Design review of the part built by this model. Coordinates are the model's own, in mm. Face numbers are marked on the shaded views. A direction names the side the tool comes from. Give positions to 0.01 mm unless a question says otherwise; leave off trailing zeros. Write each loop counter-clockwise with the first axis right and the second up, starting at its lowest first coordinate (ties: lowest second). Pieces come first, ordered by that corner, then holes.
```python
from build123d import *

# Parameters (mm, degrees)
SKETCH_1_R          = 10
SKETCH_1_R_2        = 7.5
EXTRUDE_1_DEPTH     = 80
SKETCH_2_W          = 50
SKETCH_2_H          = 20
EXTRUDE_2_DEPTH     = 70
SKETCH_3_W          = 40
SKETCH_3_H          = 20
CUT_EXTRUDE_1_DEPTH = 65
SKETCH_4_R          = 5.393818753
CUT_EXTRUDE_2_DEPTH = 159.429795178
FILLET_1_RADIUS     = 10
FILLET_1_LENGTH     = 5
FILLET_2_RADIUS     = 10
FILLET_2_LENGTH     = 5
EXTRUDE_START       = 80
SKETCH_5_R          = 7.5
EXTRUDE_3_DEPTH     = 80


with BuildPart() as part:
    # 草图1 → 凸台-拉伸1 (new body)
    with BuildSketch(Plane(origin=(0, 0, 0), x_dir=(1, 0, 0), z_dir=(0, 1, 0))):
        with Locations(Location((0, 0, 0), (0, 0, 270))):
            Circle(SKETCH_1_R)
        with Locations(Location((0, 0, 0), (0, 0, 270))):
            Circle(SKETCH_1_R_2, mode=Mode.SUBTRACT)
    extrude(amount=EXTRUDE_1_DEPTH)

    # 草图2 → 凸台-拉伸2 (add)
    with BuildSketch(Plane(origin=(0, 80, 0), x_dir=(1, 0, 0), z_dir=(0, 1, 0))):
        Rectangle(SKETCH_2_W, SKETCH_2_H)
    extrude(amount=EXTRUDE_2_DEPTH)

    # 草图3 → 切除-拉伸1 (cut)
    with BuildSketch(Plane(origin=(0, 150, 0), x_dir=(1, 0, 0), z_dir=(0, 1, 0))):
        Rectangle(SKETCH_3_W, SKETCH_3_H)
    extrude(amount=-CUT_EXTRUDE_1_DEPTH, mode=Mode.SUBTRACT)

    # 草图4 → 切除-拉伸2 (cut, through all)
    with BuildSketch(Plane.ZY.offset(25)):
        with Locations((0, 138.858219845)):
            Circle(SKETCH_4_R)
    extrude(amount=-CUT_EXTRUDE_2_DEPTH, mode=Mode.SUBTRACT)

    # 圆角1: full round fillet: the end face becomes a half cylinder, R = half its width
    fillet_1_face = Plane((-22.5, 150, 0), x_dir=(1, 0, 0), z_dir=(0, 1, 0))  # on the end face: x along it, z out of the body
    fillet_1_slab = fillet_1_face.offset(-FILLET_1_RADIUS / 2) * Box(FILLET_1_LENGTH, 2 * FILLET_1_RADIUS, FILLET_1_RADIUS, mode=Mode.PRIVATE)  # the body's end, R deep
    fillet_1_round = Plane((-22.5, 140, 0), x_dir=(0, 1, 0), z_dir=(1, 0, 0)) * Cylinder(FILLET_1_RADIUS, FILLET_1_LENGTH, mode=Mode.PRIVATE)  # its axis R under the face
    add(fillet_1_slab - fillet_1_round, mode=Mode.SUBTRACT)

    # 圆角2: full round fillet: the end face becomes a half cylinder, R = half its width
    fillet_2_face = Plane((22.5, 150, 0), x_dir=(-1, 0, 0), z_dir=(0, 1, 0))  # on the end face: x along it, z out of the body
    fillet_2_slab = fillet_2_face.offset(-FILLET_2_RADIUS / 2) * Box(FILLET_2_LENGTH, 2 * FILLET_2_RADIUS, FILLET_2_RADIUS, mode=Mode.PRIVATE)  # the body's end, R deep
    fillet_2_round = Plane((22.5, 140, 0), x_dir=(0, 1, 0), z_dir=(-1, 0, 0)) * Cylinder(FILLET_2_RADIUS, FILLET_2_LENGTH, mode=Mode.PRIVATE)  # its axis R under the face
    add(fillet_2_slab - fillet_2_round, mode=Mode.SUBTRACT)

    # 草图5 → 凸台-拉伸3 (add)
    with BuildSketch(Plane.XZ.offset(-80).offset(EXTRUDE_START)):
        Circle(SKETCH_5_R)
    extrude(amount=-EXTRUDE_3_DEPTH)

    # 草图6 → 旋转1 (revolve)
    with BuildSketch(Plane.XY):
        with BuildLine():
            Line((0, 4.111647453), (0, -10.888352547))
            ThreePointArc((0, -10.888352547), (7.5, -3.388352547), (0, 4.111647453))
        make_face()
    revolve(axis=Axis((0, 4.111647453, 0), (0, -1, 0)))


solid = part.part
```
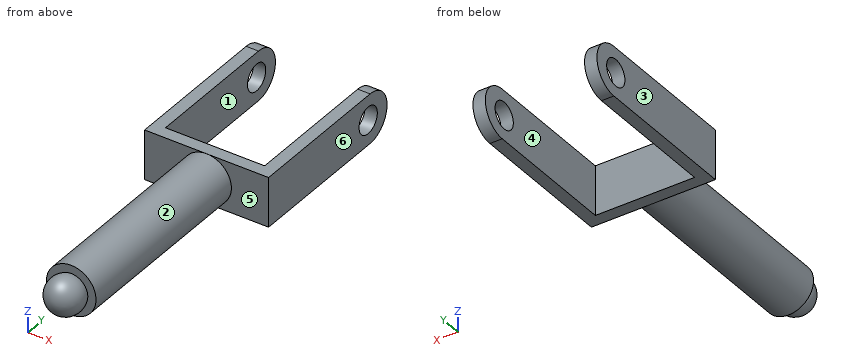
(1) Mouldability with a two-part tool opening along X and no side actions: class the marked faces 4, 5 and 6 as pulls with the +X half, pulls with the -X half, needs draft (parallel to the pull), parting line crosses it, or undercut.
Resolved:
face 4: undercut
face 5: needs draft
face 6: pulls with the +X half
(2) Consider section D-D, the plane y = 36. Give the boundary of the cut face in (x, z).
Resolved:
outline: circle Ø20 at (0, 0)
(3) Tool access review of the marked faces 1, 2 and 3: name each direction out of +Z, -Z, +X, -X, +Y, -Y from which nothing blocks a thin tool from reaching the whole face with its end or side.
Resolved:
face 1: +Z, -Z, +Y
face 2: -Y
face 3: +Z, -Z, -X, +Y, -Y
(4) Consider section B-B, the plane z = 3.75. Give the boundary of the cut face in (x, y), then the cut area to 3 significant figures.
Resolved:
outline: (-25, 80) - (-9.27, 80) - (-9.27, 0) - (-5.54, 0) arc R6.5 ccw (long way) to (5.54, 0) - (9.27, 0) - (9.27, 80) - (25, 80) - (25, 134.98) - (20, 134.98) - (20, 85) - (-20, 85) - (-20, 134.98) - (-25, 134.98) - close; (-25, 142.74) - (-20, 142.74) - (-20, 149.27) - (-25, 149.27) - close; (20, 142.74) - (25, 142.74) - (25, 149.27) - (20, 149.27) - close
area: 2,410 mm2
(5) Consider section C-C, the plane x = -2. Give the boundary of the cut face in (y, z), then the cut area to 3 significant figures.
Resolved:
outline: (0, -9.8) - (80, -9.8) - (80, -10) - (85, -10) - (85, 10) - (80, 10) - (80, 9.8) - (0, 9.8) - (0, 6.39) arc R7.23 ccw (long way) to (0, -6.39) - close
area: 1,800 mm2
(6) Clearance check with flat-ended pins moving along their axes: P1, Ø10, axis at x = -2.5, z = 2.5, coming from the -Y side; P2, Ø9.5, axis at y = 138.86, z = 0, coming from the -X side; P3, Ø5, axis at y = 20, z = 7.5, coming from the -X side; P4, Ø10, axis at x = 14.5, z = -4.5, coming from the +Y side. State where each tip first meets the part, or that it passes through.
Resolved:
P1: stops at y = -10.89
P2: passes through
P3: stops at x = -8.66
P4: stops at y = 85
(7) Consider section A-A, the plane y = 130. Give the boundary of the cut face in (x, z).
Resolved:
outline: (-25, -10) - (-20, -10) - (-20, 10) - (-25, 10) - close; (20, -10) - (25, -10) - (25, 10) - (20, 10) - close
(8) To check wall thickness, follow L1, parallel to Y at x = -23, z = 0; L2, parallel to X at y = 123.5, z = -8.5; L3, parallel to Y at x = -13, z = -3.5. State the ranges of each line that lie inside material, in increasing order.
Resolved:
L1: y = 80 to 133.46, 144.25 to 150
L2: x = -25 to -20, 20 to 25
L3: y = 80 to 85
